Study the drawing (mm; zero at the part's minimum x, y, z) and answer. Coordinates: 2 decimals unless noted, no trailing zeros. Order: outer loops, then holes, each group sorted by start corner. A loop starts at its lowest first (then second) coordinate and runs counter-clockwise, first axis right, second up. Notation, with made-up numbers: (86.5, 24.5) -> (105.5, 24.5) arc R12 cw to (105.5, 29.5) -> close; hole circle Ø1 at (23, 29.25). An arc over 180 degrees is marked (long way). Write each question's results on one line, items separated by ' | '. Start each with the question number.
(1) The part is cut by section B-B, the plane z = 0.35. Count the separate pieces of the cut face and the enclosed holes in it, then the cut area to 3 significant figures.
(2) The part is cut by section D-D, the plane y = 2.25. Give the vertices of the cut face in (x, z), then the cut area to 3 significant figures.
(3) The part is cut by section A-A, the plane y = 8. Give the vertices of the cut face in (x, z).
(4) Straight lines are drawn through the part: L1, parallel to X at y = 15.75, z = 0.7; L2, parallel to X at y = 3, z = 0.65 (1 decimal); L3, parallel to Y at x = 4.5, z = 0.85. For each, find the intervals that lie inside material, in ascending order.
(5) The part is cut by section C-C, the plane x = 9.75. Give the vertices of the cut face in (y, z).
(6) Given pin 1 (2.5 mm diameter, centred on x = 9.75, y = 15.75, fed in from -Z), flat-ended and moving along its own axis, determine where the tip first touches the part or whether it passes through.
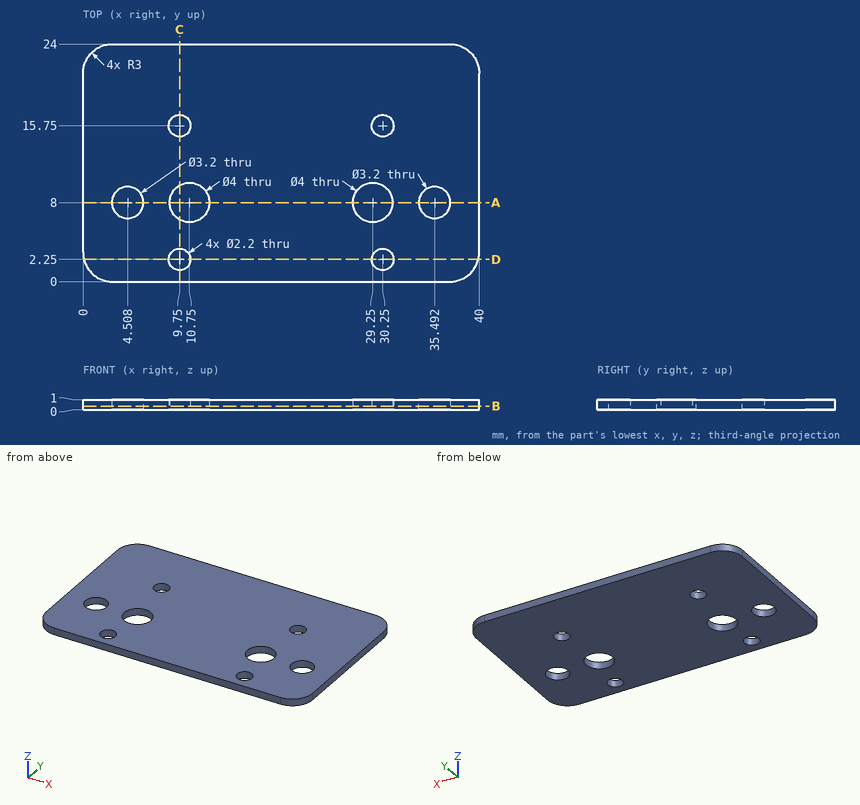
Established:
1) separate pieces: 1 | enclosed holes: 8 | area: 896 mm^2
2) outline: (0.1, 0) -> (8.65, 0) -> (8.65, 1) -> (0.1, 1) -> close; (10.85, 0) -> (29.15, 0) -> (29.15, 1) -> (10.85, 1) -> close; (31.35, 0) -> (39.9, 0) -> (39.9, 1) -> (31.35, 1) -> close | area: 35.4 mm^2
3) outline: (0, 0) -> (2.91, 0) -> (2.91, 1) -> (0, 1) -> close; (6.11, 0) -> (8.75, 0) -> (8.75, 1) -> (6.11, 1) -> close; (12.75, 0) -> (27.25, 0) -> (27.25, 1) -> (12.75, 1) -> close; (31.25, 0) -> (33.89, 0) -> (33.89, 1) -> (31.25, 1) -> close; (37.09, 0) -> (40, 0) -> (40, 1) -> (37.09, 1) -> close
4) L1: x = 0 to 8.65, 10.85 to 29.15, 31.35 to 40 | L2: x = 0 to 8.9, 10.6 to 29.4, 31.1 to 40 | L3: y = 0 to 6.4, 9.6 to 24
5) outline: (0, 0) -> (1.15, 0) -> (1.15, 1) -> (0, 1) -> close; (3.35, 0) -> (6.27, 0) -> (6.27, 1) -> (3.35, 1) -> close; (9.73, 0) -> (14.65, 0) -> (14.65, 1) -> (9.73, 1) -> close; (16.85, 0) -> (24, 0) -> (24, 1) -> (16.85, 1) -> close
6) pin 1: stops at z = 0
